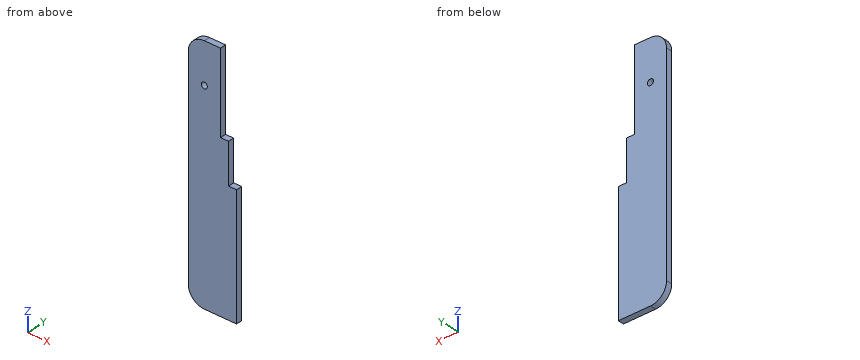
```python
from build123d import *

# Parameters (mm, degrees)
BOSS_EXTRUDE1_DEPTH              = 4.7625
FILLET1_R                        = 25.4
F_3_8_0_375_DIAMETER_HOLE1_D     = 9.525
F_3_8_0_375_DIAMETER_HOLE1_DEPTH = 11.684
F_3_8_0_375_DIAMETER_HOLE1_TIP   = 2.861598698


with BuildPart() as part:
    # Sketch1 → Boss-Extrude1 (new body, symmetric)
    with BuildSketch(Plane(origin=(0, 0, 0), x_dir=(1, 0, 0), z_dir=(0, 1, 0))):
        Polygon((0, 0), (-50.8, 0), (-50.8, 381), (25.4, 381), (25.4, 190.5), (12.7, 190.5), (12.7, 127), (0, 127), align=None)
    extrude(amount=BOSS_EXTRUDE1_DEPTH, both=True)

    # Fillet1
    fillet1_edges = [part.edges().sort_by_distance(p)[0] for p in [
        (-50.8, 0, 0),
        (-50.8, 0, -381),
    ]]
    fillet(fillet1_edges, radius=FILLET1_R)

    # 3/8 (0.375) Diameter Hole1
    with Locations(Plane(origin=(0, 4.7625, 0), x_dir=(1, 0, 0), z_dir=(0, 1, 0))):
        with Locations((-25.4, 63.5)):
            Hole(F_3_8_0_375_DIAMETER_HOLE1_D / 2, depth=F_3_8_0_375_DIAMETER_HOLE1_DEPTH)
            with Locations((0, 0, -(F_3_8_0_375_DIAMETER_HOLE1_DEPTH + F_3_8_0_375_DIAMETER_HOLE1_TIP / 2))):  # 118° drill point
                Cone(0, F_3_8_0_375_DIAMETER_HOLE1_D / 2, F_3_8_0_375_DIAMETER_HOLE1_TIP, mode=Mode.SUBTRACT)


solid = part.part
```
Model file for the job. Use its own axes, mm. Coordinates: 2 decimals unless noted, no trailing zeros. Loops run counter-clockwise (first coordinate to the right, second up) from the corner with the lowest first, then second, coordinate; pieces in that order, holes last. Notation, with made-up numbers: (6, 6) -> (50, 6) arc R15 ccw to (50, 14) -> close; hole circle Ø1 at (82.25, 74.25). An arc over 180 degrees is marked (long way). Answer as a JSON object with one key per item and string values.
Q1. Cut at C-C (x = 9). List the corners of the cut face in (y, z).
Report:
{"outline": "(-4.76, -381) -> (4.76, -381) -> (4.76, -127) -> (-4.76, -127) -> close"}
Q2. Cut at A-A (z = -63.5). List the corners of the cut face in (x, y), and give its area (3 significant figures).
Report:
{"outline": "(-50.8, -4.76) -> (-30.16, -4.76) -> (-30.16, 4.76) -> (-50.8, 4.76) -> close; (-20.64, -4.76) -> (0, -4.76) -> (0, 4.76) -> (-20.64, 4.76) -> close", "area": "393 mm2"}
Q3. Flat gauge pins, fed straight in: P1, Ø5, axis at y = 1, z = -155, coming from the +X side; P2, Ø3, axis at x = 6, y = 1, coming from the +Z side; P3, Ø4, axis at x = -38.5, y = -1.5, coming from the -Z side; P4, Ø8.5, axis at x = -25.4, z = -63.5, coming from the +Y side. Where does each tip first touch, or does it go through?
Report:
{"P1": "stops at x = 12.7", "P2": "stops at z = -127", "P3": "stops at z = -378.45", "P4": "passes through"}
Q4. Cut at B-B (y = -1.75). List the corners of the cut face in (x, z) (1 decimal), and give its area (3 significant figures).
Report:
{"outline": "(-50.8, -355.6) arc R25.4 ccw to (-25.4, -381) -> (25.4, -381) -> (25.4, -190.5) -> (12.7, -190.5) -> (12.7, -127) -> (0, -127) -> (0, 0) -> (-25.4, 0) arc R25.4 ccw to (-50.8, -25.4) -> close; hole circle Ø9.5 at (-25.4, -63.5)", "area": "24,700 mm2"}
Q5. Cut at D-D (x = -40). List the corners of the cut face in (y, z).
Report:
{"outline": "(-4.76, -376.38) -> (4.76, -376.38) -> (4.76, -4.62) -> (-4.76, -4.62) -> close"}
Q6. Probe probe 1 along X at (y, z) = (0.25, -63.5); probe 2 along Z at (x, y) = (-25.4, -1.5); probe 3 along Z at (x, y) = (12.5, 4). List the from-to ranges inside material, lowest first.
Report:
{"probe 1": "x = -50.8 to -30.16, -20.64 to 0", "probe 2": "z = -381 to -68.26, -58.74 to 0", "probe 3": "z = -381 to -127"}
